Source: CAD feature listing. Evaluate the final solid. Frame: model axes, mm. A direction names the side the tool comes from. Give positions to 0.01 mm unless a question says otherwise; leave off trailing zeros. Loops run counter-clockwise (first coordinate to the right, second up) from the corner with the lowest first, then second, coordinate; pieces in that order, holes last. Notation, with made-up numbers: (7.25, 50.25) - (49.25, 50.25) arc R28 ccw to (49.25, 88.25) - close; hole circle Ø9 at (-25, 87). An arc over 180 degrees is marked (long way). Put each result on its own line as item: value.
Autodesk Inventor part; units mm, degrees
ref_plane "Work Plane1" through (0, 46.4, 0) normal (0, 1, 0) x (1, 0, 0)
ref_plane "YZ Plane" through (0, 0, 0) normal (1, 0, 0) x (0, 1, 0)
ref_plane "XZ Plane" through (0, 0, 0) normal (0, 1, 0) x (-1, 0, 0)
sketch "Sketch1" plane through (0, 0, 0) normal (0, 1, 0) x (-1, 0, 0)
  line L0 (8, -14.25) -> (8, 14.25)
  line L1 (8, 14.25) -> (-8, 14.25)
  line L2 (-8, 14.25) -> (-8, -14.25)
  line L3 (-8, -14.25) -> (8, -14.25)
  line L4 (8, -14.25) -> (-8, 14.25) construction
  line L5 (8, 14.25) -> (-8, -14.25) construction
  point P0 (0, 0)
  dimension "d0" = 28.5
  dimension "d1" = 16
extrude "Extrusion1" add sketch "Sketch1" along normal blind 17.4
fillet "Fillet1" radius 0.5 4 edges at (-8, 8.7, 14.25) (8, 8.7, 14.25) (8, 8.7, -14.25) (-8, 8.7, -14.25)
sketch "Sketch2" plane through (0, 17.4, 0) normal (0, 1, 0) x (1, 0, 0)
  circle A0 centre (0, 0) radius 6.25
  dimension "d5" = 12.5
extrude "Extrusion2" add sketch "Sketch2" along normal blind 12
sketch "Sketch3" plane through (0, 29.4, 0) normal (0, 1, 0) x (1, 0, 0)
  circle A0 centre (0, 0) radius 2.25
  dimension "d8" = 4.5
ref_plane "Work Plane1" through (0, 46.4, 0) normal (0, 1, 0) x (1, 0, 0)
sketch "Sketch4" plane through (0, 46.4, 0) normal (0, 1, 0) x (1, 0, 0)
  circle A0 centre (0, 0) radius 3.05
  dimension "d10" = 6.1
loft "Loft1" add profiles "Sketch3", "Sketch4"
fillet "Fillet2" radius 2 1 edges at (-3.05, 46.4, 0)
chamfer "Chamfer1" distance 0.5 angle 45 1 edges at (-6.25, 29.4, 0)
thread "Thread2"
properties part number "switch"
1) Section query A-A, the plane y = 18. Output: boundary loops of the cut face in (x, z), plus the area to 3 significant figures.
Check result:
outline: circle Ø12.5 at (0, 0)
area: 123 mm²
2) Section query C-C, the plane y = 43.5. Output: boundary loops of the cut face in (x, z), plus the area to 3 significant figures.
Check result:
outline: circle Ø5.83 at (0, 0)
area: 26.7 mm²
3) Access query for faces 1 (the cylindrical face through (5.96, 23.07, 1.88)), 2 (the flat face through (2.5, 29.4, -0.1)), 3 (the flat face through (-8, 9, 0)). Directions: +Z, -Z, +X, -X, +Y, -Y. A direction counts if a zero-diameter tool reaches every point of the face in a straight line with its end or side. Return the directions, or none.
Check result:
face 1: +Y
face 2: none
face 3: +Z, -Z, -X, +Y, -Y
4) Material intervals for line 1 along Y through (x, z) = (2, 12); line 2 along Y through (x, z) = (5.5, -0.5); line 3 along X through (y, z) = (20, 3), sorted ascending. Write a range as [from, to].
Check result:
line 1: [0, 17.4]
line 2: [0, 29.4]
line 3: [-5.48, 5.48]
5) Pin query (flat end, axial travel): P1, Ø12, axis at y = 26, z = 2.5, coming from the +X side; P2, Ø2, axis at y = 21.5, z = -3, coming from the -X side; P3, Ø8, axis at x = 4.5, y = 36.5, coming from the -Z side. Return the tip coordinate at first contact, or that it passes through.
Check result:
P1: x = 6.25
P2: x = -5.92
P3: z = -2.56
6) Section query B-B, the plane x = -7. Output: boundary loops of the cut face in (y, z), plus the area to 3 significant figures.
Check result:
outline: (0, -14.25) - (17.4, -14.25) - (17.4, 14.25) - (0, 14.25) - close
area: 496 mm²
